Input: part model. Units: mm. Frame: model coordinates. Face numbers are marked on the shaded views. Give positions to 0.01 mm unless a question says otherwise; leave off trailing zeros. Loops run counter-clockwise (first coordinate to the right, second up) from the corner with the lowest first, then second, coordinate; pieces in that order, holes last. Notation, with made-up numbers: (72.25, 4) - (91.25, 4) arc R20 cw to (91.25, 36) - close; hole circle Ø2 at (66, -18). An arc over 180 degrees is marked (long way). Answer as a JSON object with one key per item and string values.
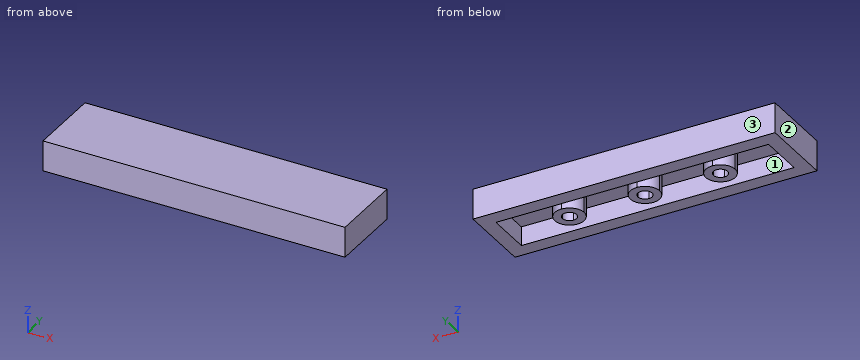
from build123d import *

# Parameters (mm, degrees)
F0_W     = 31.9
F0_H     = 7.9
F1_DEPTH = 3.2
F3_DEPTH = 2


with BuildPart() as f1:
    # F0 (on Top) → F1 (new body)
    with BuildSketch(Plane.XY):
        with Locations((4.8417709768, -0.7969564563)):
            Rectangle(F0_W, F0_H)
    extrude(amount=F1_DEPTH)

    # F2 (on face) → F3 (cut)
    with BuildSketch(Plane(origin=(0, 0, 0), x_dir=(1, 0, 0), z_dir=(0, 0, -1))):
        with BuildLine():
            Line((-3.1332290232, 3.1969564563), (-9.5582290232, 3.1969564563))
            Line((-9.5582290232, 3.1969564563), (-9.5582290232, 0.7969564563))
            Line((-9.5582290232, 0.7969564563), (-4.6832290232, 0.7969564563))
            ThreePointArc((-4.6832290232, 0.7969564563), (-4.2292445341, 1.8929719672), (-3.1332290232, 2.3469564563))
            Line((-3.1332290232, 2.3469564563), (-3.1332290232, 3.1969564563))
        make_face()
        with BuildLine():
            Line((4.8417709768, 3.1969564563), (-3.1332290232, 3.1969564563))
            Line((-3.1332290232, 3.1969564563), (-3.1332290232, 2.3469564563))
            ThreePointArc((-3.1332290232, 2.3469564563), (-2.0372135124, 1.8929719672), (-1.5832290232, 0.7969564563))
            Line((-1.5832290232, 0.7969564563), (3.2917709768, 0.7969564563))
            ThreePointArc((3.2917709768, 0.7969564563), (3.7457554659, 1.8929719672), (4.8417709768, 2.3469564563))
            Line((4.8417709768, 2.3469564563), (4.8417709768, 3.1969564563))
        make_face()
        with BuildLine():
            Line((12.8167709768, 3.1969564563), (4.8417709768, 3.1969564563))
            Line((4.8417709768, 3.1969564563), (4.8417709768, 2.3469564563))
            ThreePointArc((4.8417709768, 2.3469564563), (5.9377864876, 1.8929719672), (6.3917709768, 0.7969564563))
            Line((6.3917709768, 0.7969564563), (11.2667709768, 0.7969564563))
            ThreePointArc((11.2667709768, 0.7969564563), (11.7207554659, 1.8929719672), (12.8167709768, 2.3469564563))
            Line((12.8167709768, 2.3469564563), (12.8167709768, 3.1969564563))
        make_face()
        with BuildLine():
            Line((19.2417709768, 3.1969564563), (12.8167709768, 3.1969564563))
            Line((12.8167709768, 3.1969564563), (12.8167709768, 2.3469564563))
            ThreePointArc((12.8167709768, 2.3469564563), (13.9127864876, 1.8929719672), (14.3667709768, 0.7969564563))
            Line((14.3667709768, 0.7969564563), (19.2417709768, 0.7969564563))
            Line((19.2417709768, 0.7969564563), (19.2417709768, 3.1969564563))
        make_face()
        with BuildLine():
            Line((19.2417709768, -1.6030435437), (19.2417709768, 0.7969564563))
            Line((19.2417709768, 0.7969564563), (14.3667709768, 0.7969564563))
            ThreePointArc((14.3667709768, 0.7969564563), (13.9127864876, -0.2990590545), (12.8167709768, -0.7530435437))
            Line((12.8167709768, -0.7530435437), (12.8167709768, -1.6030435437))
            Line((12.8167709768, -1.6030435437), (19.2417709768, -1.6030435437))
        make_face()
        with BuildLine():
            Line((11.2667709768, 0.7969564563), (6.3917709768, 0.7969564563))
            ThreePointArc((6.3917709768, 0.7969564563), (5.9377864876, -0.2990590545), (4.8417709768, -0.7530435437))
            Line((4.8417709768, -0.7530435437), (4.8417709768, -1.6030435437))
            Line((4.8417709768, -1.6030435437), (12.8167709768, -1.6030435437))
            Line((12.8167709768, -1.6030435437), (12.8167709768, -0.7530435437))
            ThreePointArc((12.8167709768, -0.7530435437), (11.7207554659, -0.2990590545), (11.2667709768, 0.7969564563))
        make_face()
        with BuildLine():
            Line((3.2917709768, 0.7969564563), (-1.5832290232, 0.7969564563))
            ThreePointArc((-1.5832290232, 0.7969564563), (-2.0372135124, -0.2990590545), (-3.1332290232, -0.7530435437))
            Line((-3.1332290232, -0.7530435437), (-3.1332290232, -1.6030435437))
            Line((-3.1332290232, -1.6030435437), (4.8417709768, -1.6030435437))
            Line((4.8417709768, -1.6030435437), (4.8417709768, -0.7530435437))
            ThreePointArc((4.8417709768, -0.7530435437), (3.7457554659, -0.2990590545), (3.2917709768, 0.7969564563))
        make_face()
        with BuildLine():
            Line((-4.6832290232, 0.7969564563), (-9.5582290232, 0.7969564563))
            Line((-9.5582290232, 0.7969564563), (-9.5582290232, -1.6030435437))
            Line((-9.5582290232, -1.6030435437), (-3.1332290232, -1.6030435437))
            Line((-3.1332290232, -1.6030435437), (-3.1332290232, -0.7530435437))
            ThreePointArc((-3.1332290232, -0.7530435437), (-4.2292445341, -0.2990590545), (-4.6832290232, 0.7969564563))
        make_face()
        with BuildLine():
            Line((-3.1332290232, 0.7969564563), (-3.1332290232, 1.5469564563))
            ThreePointArc((-3.1332290232, 1.5469564563), (-3.6635591091, 1.3272865422), (-3.8832290232, 0.7969564563))
            Line((-3.8832290232, 0.7969564563), (-3.1332290232, 0.7969564563))
        make_face()
        with BuildLine():
            Line((-3.1332290232, 0.7969564563), (-3.8832290232, 0.7969564563))
            ThreePointArc((-3.8832290232, 0.7969564563), (-3.6635591091, 0.2666263705), (-3.1332290232, 0.0469564563))
            Line((-3.1332290232, 0.0469564563), (-3.1332290232, 0.7969564563))
        make_face()
        with BuildLine():
            Line((-2.3832290232, 0.7969564563), (-3.1332290232, 0.7969564563))
            Line((-3.1332290232, 0.7969564563), (-3.1332290232, 0.0469564563))
            ThreePointArc((-3.1332290232, 0.0469564563), (-2.6028989373, 0.2666263705), (-2.3832290232, 0.7969564563))
        make_face()
        with BuildLine():
            ThreePointArc((-2.3832290232, 0.7969564563), (-2.6028989373, 1.3272865422), (-3.1332290232, 1.5469564563))
            Line((-3.1332290232, 1.5469564563), (-3.1332290232, 0.7969564563))
            Line((-3.1332290232, 0.7969564563), (-2.3832290232, 0.7969564563))
        make_face()
        with BuildLine():
            Line((4.8417709768, 0.7969564563), (4.8417709768, 1.5469564563))
            ThreePointArc((4.8417709768, 1.5469564563), (4.3114408909, 1.3272865422), (4.0917709768, 0.7969564563))
            Line((4.0917709768, 0.7969564563), (4.8417709768, 0.7969564563))
        make_face()
        with BuildLine():
            ThreePointArc((5.5917709768, 0.7969564563), (5.3721010627, 1.3272865422), (4.8417709768, 1.5469564563))
            Line((4.8417709768, 1.5469564563), (4.8417709768, 0.7969564563))
            Line((4.8417709768, 0.7969564563), (5.5917709768, 0.7969564563))
        make_face()
        with BuildLine():
            Line((4.8417709768, 0.0469564563), (4.8417709768, 0.7969564563))
            Line((4.8417709768, 0.7969564563), (4.0917709768, 0.7969564563))
            ThreePointArc((4.0917709768, 0.7969564563), (4.3114408909, 0.2666263705), (4.8417709768, 0.0469564563))
        make_face()
        with BuildLine():
            Line((5.5917709768, 0.7969564563), (4.8417709768, 0.7969564563))
            Line((4.8417709768, 0.7969564563), (4.8417709768, 0.0469564563))
            ThreePointArc((4.8417709768, 0.0469564563), (5.3721010627, 0.2666263705), (5.5917709768, 0.7969564563))
        make_face()
        with BuildLine():
            Line((12.8167709768, 0.7969564563), (12.8167709768, 1.5469564563))
            ThreePointArc((12.8167709768, 1.5469564563), (12.2864408909, 1.3272865422), (12.0667709768, 0.7969564563))
            Line((12.0667709768, 0.7969564563), (12.8167709768, 0.7969564563))
        make_face()
        with BuildLine():
            ThreePointArc((13.5667709768, 0.7969564563), (13.3471010627, 1.3272865422), (12.8167709768, 1.5469564563))
            Line((12.8167709768, 1.5469564563), (12.8167709768, 0.7969564563))
            Line((12.8167709768, 0.7969564563), (13.5667709768, 0.7969564563))
        make_face()
        with BuildLine():
            Line((13.5667709768, 0.7969564563), (12.8167709768, 0.7969564563))
            Line((12.8167709768, 0.7969564563), (12.8167709768, 0.0469564563))
            ThreePointArc((12.8167709768, 0.0469564563), (13.3471010627, 0.2666263705), (13.5667709768, 0.7969564563))
        make_face()
        with BuildLine():
            Line((12.8167709768, 0.0469564563), (12.8167709768, 0.7969564563))
            Line((12.8167709768, 0.7969564563), (12.0667709768, 0.7969564563))
            ThreePointArc((12.0667709768, 0.7969564563), (12.2864408909, 0.2666263705), (12.8167709768, 0.0469564563))
        make_face()
    extrude(amount=-F3_DEPTH, mode=Mode.SUBTRACT)


solid = f1.part
Item 1: Mould query, pull axis X, two halves, no side actions, for the marked faces 1, 2 and 3. Classes: released by +X, released by -X, zero draft, split by the parting line, or undercut.
Geometry check:
{"face 1": "undercut", "face 2": "released by -X", "face 3": "zero draft"}
Item 2: Cut plane A-A (x = 9). Return loops of the section in (y, z), then the cut area to 3 significant figures.
Geometry check:
{"outline": "(-4.75, 0) - (-3.2, 0) - (-3.2, 2) - (1.6, 2) - (1.6, 0) - (3.15, 0) - (3.15, 3.2) - (-4.75, 3.2) - close", "area": "15.7 mm2"}
Item 3: Material intervals for line 1 (Y direction, x = -1, z = 1.1); line 2 (X direction, y = 0, z = 1.2); line 3 (Z direction, x = 17, y = 0.5), sorted ascending. Write a range as [from, to].
Geometry check:
{"line 1": "y = [-4.75, -3.2], [1.6, 3.15]", "line 2": "x = [-11.11, -9.56], [-4.46, -1.8], [3.51, 6.17], [11.49, 14.15], [19.24, 20.79]", "line 3": "z = [2, 3.2]"}
